Model file for the job. Use its own axes, mm. Face numbers are marked on the shaded views. Give positions to 0.01 mm unless a question says otherwise; leave off trailing zeros. Order: outer loops, then holes, each group sorted by start corner. A loop starts at its lowest first (then second) coordinate and runs counter-clockwise, first axis right, second up. Notation, with made-up numbers: (21.25, 30.5) - (37.25, 30.5) arc R21 ccw to (37.25, 43.5) - close; hole circle Ø8 at (46.5, 31). An arc over 180 degrees is marked (long way). Use CSV: the item, a comma, the result in double quotes. Start each with the question number.
(1) Band-saw the part on B-B, the plane z = -18. Give the cut face in (x, y) (3 decimals).
(2) Probe L1, parallel to X at y = 4, z = -19; L2, parallel to X at y = 0, z = -6.5 (3 decimals); L3, parallel to Y at x = -31.5, z = -15.5. List the from-to ranges inside material, lowest first.
(3) Pull direction X, two halves, no side cores. Call the marked faces 1, 2, 3 and 4: +X half, -X half, draft (parallel to the pull), parting line (faces both ways), or undercut.
(4) Band-saw the part on D-D, the plane y = -8. Give the cut face in (x, z) (3 decimals), then the cut area to 3 significant figures.
(5) Drop flat-ended pins along their axis: pin 1 Ø2 at (y, z) = (0, -56) entering from +X; pin 2 Ø4.5 at (y, z) = (-2, -17.5) entering from -X; pin 3 Ø2 at (y, z) = (5, -40.5) entering from +X. Give the stop position or say it passes through.
(6) Band-saw the part on A-A, the plane y = 0. Give the cut face in (x, z) (3 decimals), then the cut area to 3 significant figures.
(7) Band-saw the part on C-C, the plane x = 0. Give the cut face in (y, z) (3 decimals), then the cut area to 3 significant figures.
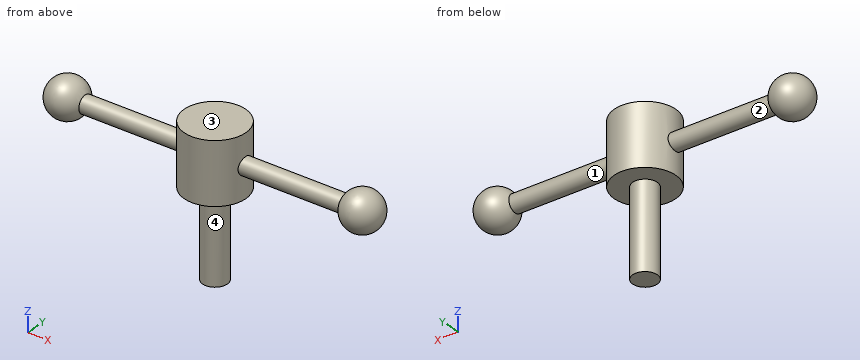
from build123d import *

# Parameters (mm, degrees)
F0_R     = 15.875
F0_R_2   = 6.35
F1_DEPTH = 31.75
F2_DEPTH = 76.2
F3_R     = 4.445
F4_DEPTH = 76.2


with BuildPart() as f1:
    # F0 (on Top) → F1 (new body)
    with BuildSketch(Plane.XY):
        Circle(F0_R)
        Circle(F0_R_2, mode=Mode.SUBTRACT)
        Circle(F0_R_2)
    extrude(amount=-F1_DEPTH)

    # F0 (on Top) → F2 (join)
    with BuildSketch(Plane.XY):
        Circle(F0_R_2)
    extrude(amount=-F2_DEPTH)

    # F3 (on Right) → F4 (join, symmetric)
    with BuildSketch(Plane.YZ):
        with Locations((0, -15.875)):
            Circle(F3_R)
    extrude(amount=F4_DEPTH, both=True)

    # F5 (on face) → F6 (revolve)
    with BuildSketch(Plane.YZ.offset(76.2)):
        with BuildLine():
            Line((-10.16, -15.875), (10.16, -15.875))
            ThreePointArc((10.16, -15.875), (0, -5.715), (-10.16, -15.875))
        make_face()
    revolve(axis=Axis((76.2, 10.16, -15.875), (0, 1, 0)))

    # F7 (on face) → F8 (revolve)
    with BuildSketch(Plane(origin=(-76.2, 0, 0), x_dir=(0, -1, 0), z_dir=(-1, 0, 0))):
        with BuildLine():
            Line((4.445, -15.875), (10.16, -15.875))
            ThreePointArc((10.16, -15.875), (0, -5.715), (-10.16, -15.875))
            Line((-10.16, -15.875), (-4.445, -15.875))
            ThreePointArc((-4.445, -15.875), (0, -11.43), (4.445, -15.875))
        make_face()
    revolve(axis=Axis((-76.2, -10.16, -15.875), (0, -1, 0)))


solid = f1.part
Answer block:
1,outline,"(-67.064, -3.904) - (-15.387, -3.904) arc R15.875 ccw to (15.387, -3.904) - (67.064, -3.904) arc R9.935 ccw (long way) to (67.064, 3.904) - (15.387, 3.904) arc R15.875 ccw to (-15.387, 3.904) - (-67.064, 3.904) arc R9.935 ccw (long way) to start; hole (-76.2, -3.904) - (-76.2, 3.904) arc R3.904 ccw to start"
2,L1,"x = -85 to -67.4, -15.36 to 15.36, 67.4 to 85"
2,L2,"x = -80.116 to -72.284, -15.875 to 15.875, 72.284 to 80.116"
2,L3,"y = -4.43 to 4.43"
3,face 1,"undercut"
3,face 2,"undercut"
3,face 3,"draft"
3,face 4,"parting line"
4,outline,"circle Ø12.526 at (-76.2, -15.875); (-13.712, -31.75) - (13.712, -31.75) - (13.712, 0) - (-13.712, 0) - close; circle Ø12.526 at (76.2, -15.875)"
4,area,"1,120 mm2"
5,pin 1,"stops at x = 6.35"
5,pin 2,"stops at x = -86.35"
5,pin 3,"stops at x = 4.93"
6,outline,"(-67.064, -20.32) - (-15.875, -20.32) - (-15.875, -31.75) - (-6.35, -31.75) - (-6.35, -76.2) - (6.35, -76.2) - (6.35, -31.75) - (15.875, -31.75) - (15.875, -20.32) - (67.064, -20.32) arc R10.16 ccw (long way) to (67.064, -11.43) - (15.875, -11.43) - (15.875, 0) - (-15.875, 0) - (-15.875, -11.43) - (-67.064, -11.43) arc R10.16 ccw (long way) to start; hole (-76.2, -20.32) - (-76.2, -11.43) arc R4.445 ccw to start"
6,area,"3,090 mm2"
7,outline,"(-15.875, -31.75) - (-6.35, -31.75) - (-6.35, -76.2) - (6.35, -76.2) - (6.35, -31.75) - (15.875, -31.75) - (15.875, 0) - (-15.875, 0) - close"
7,area,"1,570 mm2"
